Input: part model. Units: mm. Frame: model coordinates. Give positions to 0.01 mm unless a question says otherwise; leave off trailing zeros. Loops run counter-clockwise (first coordinate to the right, second up) from the corner with the lowest first, then second, coordinate; pieces in that order, holes last. Notation, with made-up numbers: (44, 29.25) -> (71, 29.25) arc R13 cw to (71, 48.25) -> close; hole circle Ø6 at (53, 1.25). An arc over 180 degrees is marked (long way). Answer as a JSON object with one key per item and string values. Group by question number.
```python
from build123d import *

# Parameters (mm, degrees)
F0_W     = 139.7
F0_H     = 27.94
F1_DEPTH = 355.6
F2_SIZE  = 27.93999
F3_W     = 38.1
F3_H     = 355.6
F4_DEPTH = 3.175
F6_DEPTH = 38.1


# Not quite as in the source:
# - a fillet or chamfer is up to 0.001 mm smaller than in the source, because OpenCascade refuses the exact size


with BuildPart() as f1:
    # F0 (on Top) → F1 (new body)
    with BuildSketch(Plane.XY):
        with Locations((69.85, -13.97)):
            Rectangle(F0_W, F0_H)
    extrude(amount=F1_DEPTH)

    # F2 (size 27.94 in the source; OpenCascade refuses exactly that, so slightly less here)
    f2_edges = [f1.edges().sort_by_distance(p)[0] for p in [
        (69.85, -27.94, 355.6),
    ]]
    chamfer(f2_edges, length=F2_SIZE)

    # F3 (on face) → F4 (cut)
    with BuildSketch(Plane.XZ.offset(27.94)):
        with Locations((69.85, 177.8)):
            Rectangle(F3_W, F3_H)
    extrude(amount=-F4_DEPTH, mode=Mode.SUBTRACT)

    # F5 (on face) → F6 (cut)
    with BuildSketch(Plane(origin=(0, 0, 0), x_dir=(-1, 0, 0), z_dir=(0, 1, 0))):
        Polygon((0, 327.66), (0, 355.6), (-27.94, 355.6), align=None)
    extrude(amount=-F6_DEPTH, mode=Mode.SUBTRACT)


solid = f1.part
```
Q1. Section A-A on y = -18.5. Return the cut outline in (x, z), then the cut area to 3 significant figures.
Q2. Section B-B on z = 172. Return the cut outline in (x, y) (3 decimals), then the cut area to 3 significant figures.
Q3. Pull-direction query (X, two-part tool) for faces 1 (the face through (0, -14, 162)), 2 (the face through (70, -24.765, 168)), 3 (the face through (114, -27.94, 162)); classes: +X half, -X half, draft (parallel to the pull), parting line (faces both ways), or undercut.
Q4. Ray query, probe 1 along X at (y, z) = (-25.75, 131.5); probe 2 along Y at (x, z) = (54.5, 327.5) (3 decimals); probe 3 along Z at (x, y) = (107.5, -25.5). Return the intervals inside material, ascending.
Q5. Pin query (flat end, axial travel): pin 1 Ø10 at (x, y) = (28, -16.5) entering from +Z; pin 2 Ø5 at (x, z) = (75.5, 239.5) entering from -Y (3 decimals); pin 3 Ø1 at (x, y) = (40, -7) entering from +Z. Return the tip coordinate at first contact, or that it passes through.
Numbers:
{
 "1": {"outline": "(0, 0) -> (139.7, 0) -> (139.7, 337.1) -> (9.44, 337.1) -> (0, 327.66) -> close", "area": "47,000 mm²"},
 "2": {"outline": "(0, -27.94) -> (50.8, -27.94) -> (50.8, -24.765) -> (88.9, -24.765) -> (88.9, -27.94) -> (139.7, -27.94) -> (139.7, 0) -> (0, 0) -> close", "area": "3,780 mm²"},
 "3": {"face 1": "-X half", "face 2": "undercut", "face 3": "draft"},
 "4": {"probe 1": "x = 0 to 50.8, 88.9 to 139.7", "probe 2": "y = -24.765 to 0", "probe 3": "z = 0 to 330.1"},
 "5": {"pin 1": "stops at z = 344.1", "pin 2": "stops at y = -24.765", "pin 3": "stops at z = 349.1"}
}
